Design review of the part built by this model. Coordinates are the model's own, in mm. A direction names the side the tool comes from. Round coordinates to 2 decimals unless told otherwise and drop trailing zeros. Write each loop counter-clockwise with the first axis right and the second up, starting at its lowest first coordinate (ties: lowest second). Pieces come first, ordered by that corner, then holes. Notation, with made-up numbers: M 48,35.5 L 104,35.5 A20 cw 104,44.5 Z; hole C 4,77 d6. An arc over 180 degrees is marked long. Use CSV: the item, a comma, the result in double quotes.
Autodesk Inventor part; units mm, degrees
ref_plane "YZ Plane" through (0, 0, 0) normal (1, 0, 0) x (0, 1, 0)
ref_plane "XZ Plane" through (0, 0, 0) normal (0, 1, 0) x (-1, 0, 0)
ref_plane "XY Plane" through (0, 0, 0) normal (0, 0, 1) x (1, 0, 0)
sketch "Sketch1" plane through (0, 0, 0) normal (0, 0, 1) x (1, 0, 0)
  line L0 (-15.6216, 9.2219) -> (35.1784, 9.2219)
  line L1 (35.1784, 9.2219) -> (35.1784, -16.1781)
  line L2 (35.1784, -16.1781) -> (-15.6216, -16.1781)
  line L3 (-15.6216, -16.1781) -> (-15.6216, 9.2219)
  line L4 (-14.0341, 7.6344) -> (33.5909, 7.6344)
  line L5 (33.5909, 7.6344) -> (33.5909, -14.5906)
  line L6 (33.5909, -14.5906) -> (-14.0341, -14.5906)
  line L7 (-14.0341, -14.5906) -> (-14.0341, 7.6344)
  point P0 (0, 0)
  dimension "d0" = 50.8
  dimension "d1" = 25.4
  dimension "d2" = 1.5875
  dimension "d3" = 1.5875
  dimension "d4" = 1.5875
  dimension "d5" = 1.5875
extrude "Extrusion1" add sketch "Sketch1" along normal blind 95.25
sketch "Sketch2" plane through (-15.6216, 9.2219, 0) normal (0, 1, 0) x (1, 0, 0)
  circle A0 centre (25.4, -47.625) radius 9.525
  line L0 (0, 0) -> (0, -95.25)
  line L1 (50.8, 0) -> (0, 0)
  line L2 (12.7, 0) -> (38.1, 0)
  line L3 (38.1, 0) -> (38.1, -25.4)
  line L4 (38.1, -25.4) -> (12.7, -25.4)
  line L5 (12.7, -25.4) -> (12.7, 0)
  line L6 (1.5875, -95.25) -> (49.2125, -95.25)
  line L7 (12.7, -95.25) -> (38.1, -95.25)
  line L8 (38.1, -95.25) -> (38.1, -69.85)
  line L9 (38.1, -69.85) -> (12.7, -69.85)
  line L10 (12.7, -69.85) -> (12.7, -95.25)
  point P0 (15.6216, 0)
  point P1 (25.4, -25.4)
  dimension "d8" = 19.05
  dimension "d9" = 25.4
  dimension "d10" = 47.625
  dimension "d13" = 25.4
  dimension "d14" = 25.4
  dimension "d15" = 25.4
  dimension "d16" = 25.4
  dimension "d25" = 95.25
extrude "Extrusion2" cut sketch "Sketch2" against normal blind 116.84
sketch "Sketch3" plane through (35.1784, -16.1781, 0) normal (1, 0, 0) x (0, 0, -1)
  circle A0 centre (-12.7, 12.7) radius 3.175
  line L0 (0, 25.4) -> (-95.25, 25.4)
  circle A1 centre (-82.55, 12.7) radius 3.175
  line L1 (-95.25, 0) -> (-95.25, 25.4)
  point P0 (0, 16.1781)
  dimension "d17" = 6.35
  dimension "d18" = 12.7
  dimension "d19" = 12.7
  dimension "d20" = 6.35
  dimension "d21" = 12.7
  dimension "d22" = 12.7
extrude "Extrusion3" cut sketch "Sketch3" against normal through all
equation "\"d3\" = d2"
equation "\"d4\" = d2"
equation "\"d5\" = d2"
equation "\"d10\" = 0.5 * d25"
properties part number "Diff Top Bar"
1) Add section B-B on y = 2. Write out the cut boundary in (x, z), then the cut area to 3 significant figures.
Answers:
outline,"M -15.62,0 L -14.03,0 L -14.03,95.25 L -15.62,95.25 Z; M 33.59,0 L 35.18,0 L 35.18,95.25 L 33.59,95.25 Z"
area,"302 mm²"
2) Add section A-A on z = 82.55. Write out the cut boundary in (x, y).
Answers:
outline,"M -15.62,-16.18 L -2.92,-16.18 L -2.92,-14.59 L -14.03,-14.59 L -14.03,-6.65 L -15.62,-6.65 Z; M -15.62,-0.3 L -14.03,-0.3 L -14.03,7.63 L -2.92,7.63 L -2.92,9.22 L -15.62,9.22 Z; M 22.48,-16.18 L 35.18,-16.18 L 35.18,-6.65 L 33.59,-6.65 L 33.59,-14.59 L 22.48,-14.59 Z; M 22.48,7.63 L 33.59,7.63 L 33.59,-0.3 L 35.18,-0.3 L 35.18,9.22 L 22.48,9.22 Z"
3) Wall thickness on line 1 along Y through (x, z) = (16, 65.5); line 2 along X through (y, z) = (-13.5, 26); line 3 along Y through (x, z) = (-14.45, 82.55): over which ranges is each line inside the solid? List them lowest first. Write a range as [from, to].
Answers:
line 1,"[-16.18, -14.59], [7.63, 9.22]"
line 2,"[-15.62, -14.03], [33.59, 35.18]"
line 3,"[-16.18, -6.65], [-0.3, 9.22]"
4) Add section C-C on x = 9. Write out the cut boundary in (y, z), then the cut area to 3 significant figures.
Answers:
outline,"M -16.18,25.4 L -14.59,25.4 L -14.59,38.13 L -16.18,38.13 Z; M -16.18,57.12 L -14.59,57.12 L -14.59,69.85 L -16.18,69.85 Z; M 7.63,25.4 L 9.22,25.4 L 9.22,38.13 L 7.63,38.13 Z; M 7.63,57.12 L 9.22,57.12 L 9.22,69.85 L 7.63,69.85 Z"
area,"80.8 mm²"
5) Machinability: for faces 1 (the face through (-15.622, -4, 47)), 2 (the face through (-14.034, -4, 47)), which of the approach directions +Z, -Z, +X, -X, +Y, -Y give a long, thin tool a straight path to every point of the face, cutting with its end or side? Answer none if there is none.
Answers:
face 1,"+Z, -Z, -X, +Y, -Y"
face 2,"+Z, -Z"
6) The part is to be moulded in two halves that separate along Y. For faces 3 (the face through (7.714, 8.439, 56.923)), 4 (the face through (10, -14.591, 36)), 5 (the face through (9, 9.222, 36)), say which applies: released by +Y, released by -Y, zero draft, split by the parting line, or undercut.
Answers:
face 3,"zero draft"
face 4,"undercut"
face 5,"released by +Y"
7) Add section D-D on y = -5.5. Write out the cut boundary in (x, z).
Answers:
outline,"M -15.62,0 L -14.03,0 L -14.03,10.25 L -15.62,10.25 Z; M -15.62,15.15 L -14.03,15.15 L -14.03,80.1 L -15.62,80.1 Z; M -15.62,85 L -14.03,85 L -14.03,95.25 L -15.62,95.25 Z; M 33.59,0 L 35.18,0 L 35.18,10.25 L 33.59,10.25 Z; M 33.59,15.15 L 35.18,15.15 L 35.18,80.1 L 33.59,80.1 Z; M 33.59,85 L 35.18,85 L 35.18,95.25 L 33.59,95.25 Z"
8) For pin 1 Ø5 at (y, z) = (-3.48, 82.55) entering from -X; pin 2 Ø0.8 at (x, y) = (13, 8.5) entering from +Z; pin 3 Ø0.8 at (x, y) = (4.5, -15) entering from -Z, all flat-tipped, find the tip position at first contact; note any pin that passes through.
Answers:
pin 1,"through"
pin 2,"z = 69.85"
pin 3,"z = 25.4"
